from build123d import *

# Parameters (mm, degrees)
FILETE1_R     = 2
CHANFRO1_SIZE = 0.5


with BuildPart() as part:
    # Esboço1 → Revolução1 (revolve)
    with BuildSketch(Plane.XY, mode=Mode.PRIVATE) as revolu_o1_sk:
        Polygon((0, 57.501605759), (12.5, 57.501605759), (12.5, 53.501605759), (6.95, 53.501605759), (6.95, 40.101605759), (5, 40.101605759), (5, 16.101605759), (0, 16.101605759), align=None)
    revolve(revolu_o1_sk.sketch.rotate(Axis((0, -51.285215947, 0), (0, 1, 0)), 90), axis=Axis((0, -51.285215947, 0), (0, 1, 0)))

    # Filete1
    filete1_edges = [part.edges().sort_by_distance(p)[0] for p in [
        (0, 53.501605759, 12.5),
        (0, 57.501605759, 12.5),
    ]]
    fillet(filete1_edges, radius=FILETE1_R - 0.0001)  # a hair under: the kernel refuses the full size

    # Chanfro1
    chanfro1_edges = [part.edges().sort_by_distance(p)[0] for p in [
        (0, 16.101605759, 5),
    ]]
    chamfer(chanfro1_edges, length=CHANFRO1_SIZE)


solid = part.part
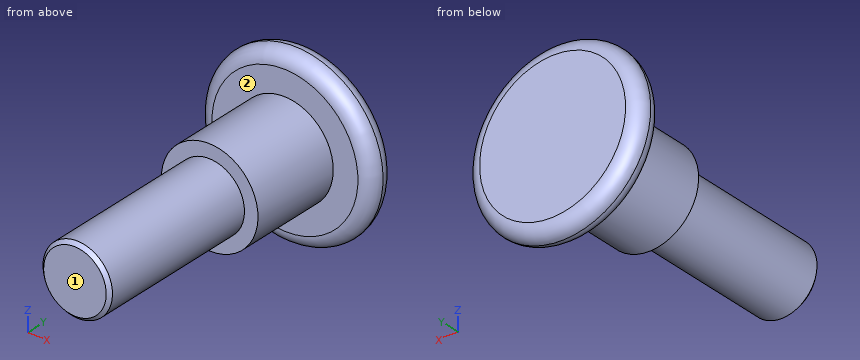
The model under review builds one solid part; all positions refer to its coordinate system, in mm. Face numbers are marked on the shaded views. A direction names the side the tool comes from. Give positions to 0.01 mm unless a question says otherwise; leave off trailing zeros. Write each loop counter-clockwise with the first axis right and the second up, starting at its lowest first coordinate (ties: lowest second). Pieces come first, ordered by that corner, then holes. Notation, with made-up numbers: M 10.25,4.25 L 53.25,4.25 A20 cw 53.25,18.25 Z; hole C -22,17 d8. An arc over 180 degrees is marked long. One line per question, with ' | ' between items. Start each with the question number.
Item 1: For pin 1 (5 mm diameter, centred on x = -1.5, y = 50, fed in from -Z); pin 2 (2 mm diameter, centred on x = 1, z = -9.5, fed in from -Y); pin 3 (4 mm diameter, centred on x = 9, y = 48, fed in from -Z), all flat-tipped, find the tip position at first contact; note any pin that passes through.
Item 2: For the marked faces 1 and 2, list the 3-axis set-ups (+Z, -Z, +X, -X, +Y, -Y) from which the entire face can be reached by the end or side of a thin tool; tool diameter is ignored.
Item 3: Wall thickness on line 1 (Y direction, x = 5.25, z = -8.5); line 2 (Y direction, x = -2, z = -5.25); line 3 (X direction, y = 40.5, z = 0.25): over which ranges is each line inside the solid? List them lowest first. Write a range as from..to.
Item 4: We need section C-C on y = 21.5. Write out the cut boundary in (x, z), plus the area to 3 significant figures.
Results found:
1) pin 1: stops at z = -6.95 | pin 2: stops at y = 53.5 | pin 3: passes through
2) face 1: +Z, -Z, +X, -X, -Y | face 2: -Y
3) line 1: y = 53.5..57.5 | line 2: y = 40.1..57.5 | line 3: x = -6.95..6.95
4) outline: C 0,0 d10 | area: 78.5 mm2
